Here's the drawing with two shaded views (mm, measured from the low corner). I have some questions. Coordinates: 2 decimals unless noted, no trailing zeros. Loops run counter-clockwise (first coordinate to the right, second up) from the corner with the lowest first, then second, coordinate; pieces in that order, holes last. Notation, with made-up numbers: M 6.25,87.25 L 40.25,87.25 A24 ccw 40.25,111.25 Z; hole C 17,-22.5 d8. An arc over 180 degrees is marked long. Return JSON: item names as keys, results as strings. Group by question number.
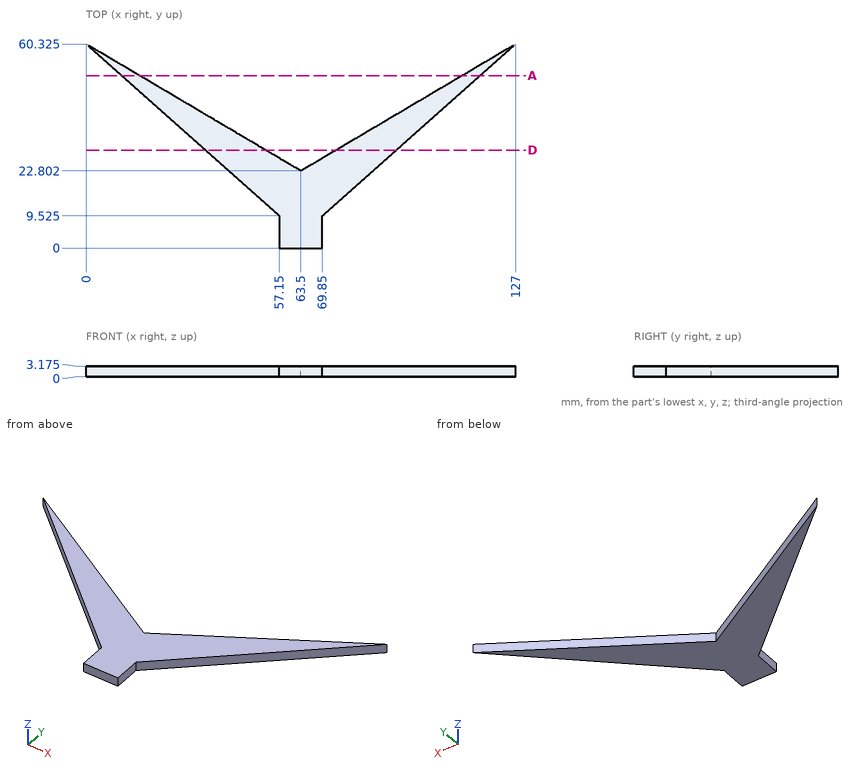
(1) If I drill on L1, parallel to X at y = 50.5, z = 1 (1 decimal); L2, parallel to X at y = 8, z = 2.2; L3, parallel to X at y = 44, z = 1 (1 decimal), over which ranges is the centre line in solid material (lowest first)? Write a range as [from, to].
(2) Imagine slicing it at A-A, the plane y = 51. Write out the boundary of the cut face in (x, z) (1 decimal).
(3) Will these pins go through, and if not, where does the flat tip stop? P1, Ø1, axis at y = 6.5, z = 2.5, coming from the -X side; P2, Ø1, axis at x = 21.5, z = 0.5, coming from the -Y side; P3, Ø1.6, axis at y = 6.5, z = 2, coming from the +X side.
(4) Imagine slicing it at D-D, the plane y = 29. Write out the boundary of the cut face in (x, z) (1 decimal), then the cut area to 3 significant figures.
Checks:
{
 "1": {"L1": "[11.1, 16.6], [110.4, 115.9]", "L2": "[57.15, 69.85]", "L3": "[18.4, 27.6], [99.4, 108.6]"},
 "2": {"outline": "M 10.5,0 L 15.8,0 L 15.8,3.2 L 10.5,3.2 Z; M 111.2,0 L 116.5,0 L 116.5,3.2 L 111.2,3.2 Z"},
 "3": {"P1": "x = 57.15", "P2": "y = 40.77", "P3": "x = 69.85"},
 "4": {"outline": "M 35.2,0 L 53,0 L 53,3.2 L 35.2,3.2 Z; M 74,0 L 91.8,0 L 91.8,3.2 L 74,3.2 Z", "area": "113 mm²"}
}
